from build123d import *

# Parameters (mm, degrees)
SKETCH_1_R          = 3.75
EXTRUDE_1_DEPTH     = 3
SKETCH_2_R          = 2
EXTRUDE_2_DEPTH     = 15
CHAMFER_1_SIZE      = 0.5
CUT_EXTRUDE_1_DEPTH = 1


with BuildPart() as part:
    # 草图1 → 凸台-拉伸1 (new body)
    with BuildSketch(Plane(origin=(0, 0, 0), x_dir=(1, 0, 0), z_dir=(0, 1, 0))):
        with Locations(Location((0, 0, 0), (0, 0, 270))):
            Circle(SKETCH_1_R)
    extrude(amount=EXTRUDE_1_DEPTH)

    # 草图2 → 凸台-拉伸2 (add)
    with BuildSketch(Plane(origin=(0, 3, 0), x_dir=(1, 0, 0), z_dir=(0, 1, 0))):
        with Locations(Location((0, 0, 0), (0, 0, 270))):
            Circle(SKETCH_2_R)
    extrude(amount=EXTRUDE_2_DEPTH)

    # 倒角1
    chamfer_1_edges = [part.edges().sort_by_distance(p)[0] for p in [
        (0, 0, -3.75),
        (0, 3, -3.75),
    ]]
    chamfer(chamfer_1_edges, length=CHAMFER_1_SIZE)

    # 草图3 → 切除-拉伸1 (cut)
    with BuildSketch(Plane.XZ):
        Polygon((0, -2.886751346), (2.5, -1.443375673), (2.5, 1.443375673), (0, 2.886751346), (-2.5, 1.443375673), (-2.5, -1.443375673), align=None)
    extrude(amount=-CUT_EXTRUDE_1_DEPTH, mode=Mode.SUBTRACT)


solid = part.part
Can you work these out from the model? Positions are in its coordinate system, mm. A direction names the side the tool comes from. Coordinates: 2 decimals unless noted, no trailing zeros. Order: outer loops, then holes, each group sorted by start corner. A loop starts at its lowest first (then second) coordinate and runs counter-clockwise, first axis right, second up. Notation, with made-up numbers: M -38.75,-11 L 6.25,-11 A19 cw 6.25,7 Z; hole C 31.25,-32.5 d11. An arc over 180 degrees is marked long. Write item = value, one per line.
(1) For faces 5 (the face through (1.267, 0.493, 2.155)), 6 (the face through (-2, 3, 1)), 7 (the face through (0.165, 1.486, -3.746)), which set-ups out of +Z, -Z, +X, -X, +Y, -Y let a thin tool reach every point of the face, with its end or its side?
Results are:
face_5 = -Y
face_6 = +Y
face_7 = +Y, -Y
(2) Suppose I cut it at B-B on y = 13. Please give me the cut outline in (x, z), plus the area to 3 significant figures.
Results are:
outline = C 0,0 d4
area = 12.6 mm2
(3) For pin 1 Ø3 at (x, y) = (-1, 10) entering from +Z; pin 2 Ø4 at (y, z) = (13.5, -2) entering from -X; pin 3 Ø1.5 at (y, z) = (4, 3) entering from -X; pin 4 Ø4 at (y, z) = (8.5, 1.5) entering from +X, each with a flat end and sliding along its axis, tell me the tip position at first contact or that it passes through.
Results are:
pin_1 = 2
pin_2 = -2
pin_3 = through
pin_4 = 2
(4) Suppose I cut it at A-A on z = 0. Please give me the cut outline in (x, y), plus the area to 3 significant figures.
Results are:
outline = M -3.75,0.5 L -3.25,0 L -2.5,0 L -2.5,1 L 2.5,1 L 2.5,0 L 3.25,0 L 3.75,0.5 L 3.75,2.5 L 3.25,3 L 2,3 L 2,18 L -2,18 L -2,3 L -3.25,3 L -3.75,2.5 Z
area = 77.0 mm2
(5) I need wall thicknesses on line 1 along Y through (x, z) = (1, -3); line 2 along Y through (x, z) = (-0.75, 0.75); line 3 along X through (y, z) = (14.75, -1.5). Which ranges of each line are inside material? Lowest first, please. Write a range as [from, to].
Results are:
line_1 = [0, 3]
line_2 = [1, 18]
line_3 = [-1.32, 1.32]
(6) If we mould it in two halves opening along X, with no side actions, what happens to faces 1 (the face through (-1.267, 0.493, -2.155)), 2 (the face through (-2, 0, -2)), 3 (the face through (-2, 10, 0)), 4 (the face through (0, 1, 0))? For each: pulls with the +X half, pulls with the -X half, needs draft (parallel to the pull), parting line crosses it, or undercut.
Results are:
face_1 = undercut
face_2 = needs draft
face_3 = parting line crosses it
face_4 = undercut
